For this review, take the finished solid that the model builds, in its own axes (mm). A direction names the side the tool comes from. Coordinates: 2 decimals unless noted, no trailing zeros. Order: outer loops, then holes, each group sorted by start corner. A loop starts at its lowest first (then second) coordinate and runs counter-clockwise, first axis right, second up.
from build123d import *

# Parameters (mm, degrees)
ESBO_O1_W                                           = 170
ESBO_O1_H                                           = 42
ESBO_O1_R                                           = 6
ESBO_O1_R_2                                         = 4
RESSALTO_EXTRUS_O1_DEPTH                            = 10
REBAIXO_PARA_PARAFUSO_COM_CABE_A_PANELA_D           = 3.4
REBAIXO_PARA_PARAFUSO_COM_CABE_A_PANELA_CBORE_D     = 7
REBAIXO_PARA_PARAFUSO_COM_CABE_A_PANELA_CBORE_DEPTH = 2.4
ESBO_O7_W                                           = 42.5
ESBO_O7_H                                           = 46.397828282
CORTE_EXTRUS_O2_DEPTH                               = 1.5
FILETE1_R                                           = 5


with BuildPart() as part:
    # Esboço1 → Ressalto-extrusão1 (new body)
    with BuildSketch(Plane(origin=(0, 0, 0), x_dir=(1, 0, 0), z_dir=(0, 1, 0))):
        Rectangle(ESBO_O1_W, ESBO_O1_H)
        with Locations(Location((-57.5, 0, 0), (0, 0, 270))):
            Circle(ESBO_O1_R, mode=Mode.SUBTRACT)
        with Locations(Location((57.5, 0, 0), (0, 0, 270))):
            Circle(ESBO_O1_R, mode=Mode.SUBTRACT)
        with Locations(Location((0, 0, 0), (0, 0, 270))):
            Circle(ESBO_O1_R_2, mode=Mode.SUBTRACT)
    extrude(amount=RESSALTO_EXTRUS_O1_DEPTH)

    # Esboço2 → Furo roscado de M51 (revolve, cut)
    with BuildSketch(Plane(origin=(85, 5, -1), x_dir=(0, 0, -1), z_dir=(0, 1, 0))):
        Polygon((0, 0), (0, 15.2618073), (2.1, 14), (2.1, 0), align=None)
    furo_roscado_de_m51 = revolve(axis=Axis((91.35, 5, -1), (-1, 0, 0)), mode=Mode.SUBTRACT)

    # Espelhar1: Furo roscado de M51 across plane
    add(furo_roscado_de_m51.mirror(Plane(origin=(0, 0, 0), x_dir=(0, 0, 1), z_dir=(1, 0, 0))), mode=Mode.SUBTRACT)

    # Rebaixo para parafuso com cabeça panela de M31 (through all)
    with Locations(Plane(origin=(0, 0, 0), x_dir=(-1, 0, 0), z_dir=(0, -1, 0))):
        with Locations((-15.5, 15.5), (15.5, 15.5), (-15.5, -15.5), (15.5, -15.5)):
            CounterBoreHole(REBAIXO_PARA_PARAFUSO_COM_CABE_A_PANELA_D / 2, REBAIXO_PARA_PARAFUSO_COM_CABE_A_PANELA_CBORE_D / 2, REBAIXO_PARA_PARAFUSO_COM_CABE_A_PANELA_CBORE_DEPTH)

    # Esboço7 → Corte-extrusão2 (cut)
    with BuildSketch(Plane(origin=(0, 10, 0), x_dir=(1, 0, 0), z_dir=(0, 1, 0))):
        with Locations((0, -0.001085859)):
            Rectangle(ESBO_O7_W, ESBO_O7_H)
    extrude(amount=-CORTE_EXTRUS_O2_DEPTH, mode=Mode.SUBTRACT)

    # Filete1
    filete1_edges = [part.edges().sort_by_distance(p)[0] for p in [
        (85, 5, 21),
        (-85, 5, 21),
        (-85, 5, -21),
        (85, 5, -21),
    ]]
    fillet(filete1_edges, radius=FILETE1_R)


solid = part.part
1. Clearance check with flat-ended pins moving along their axes: pin 1 Ø6.5 at (x, z) = (0, 0) entering from +Y; pin 2 Ø2.5 at (y, z) = (5, -1) entering from +X; pin 3 Ø4 at (x, z) = (-15.5, -15.5) entering from -Y; pin 4 Ø12.5 at (x, z) = (-1, 4.5) entering from +Y. State where each tip first meets the part, or that it passes through.
Answer below:
pin 1: passes through
pin 2: stops at x = 70.49
pin 3: stops at y = 2.4
pin 4: stops at y = 8.5
2. Machinability: for faces 1 (the face through (-84, 5, -19)), 2 (the face through (78.1, 7.05, -0.54)), 3 (the face through (12.16, 1.18, -16.55)), which of the approach directions +Z, -Z, +X, -X, +Y, -Y give a long, thin tool a straight path to every point of the face, cutting with its end or side? Answer none if there is none.
Answer below:
face 1: -Z, -X, +Y, -Y
face 2: +X
face 3: -Y
3. Take a section at C-C, the plane z = -10.5. Give the boundary of the cut face in (x, y).
Answer below:
outline: (-85, 0) - (85, 0) - (85, 10) - (21.25, 10) - (21.25, 8.5) - (-21.25, 8.5) - (-21.25, 10) - (-85, 10) - close
4. The part is to be moulded in two halves that separate along X. For faces 4 (the face through (-14.7, 5.5, -14)), 5 (the face through (-1, 5, -21)), 6 (the face through (-18.84, 1.18, -16.55)), 7 (the face through (-84, 5, 19)), say which applies: +X half, -X half, draft (parallel to the pull), parting line (faces both ways), or undercut.
Answer below:
face 4: undercut
face 5: draft
face 6: undercut
face 7: -X half
5. Take a section at B-B, the plane x = 57.5. Give the boundary of the cut face in (y, z).
Answer below:
outline: (0, -21) - (10, -21) - (10, -6) - (0, -6) - close; (0, 6) - (10, 6) - (10, 21) - (0, 21) - close
6. To check wall thickness, follow L1, parallel to X at y = 4.25, z = -15.5; L2, parallel to X at y = 1.6, z = -15.5; L3, parallel to Z at x = -15.5, y = 4.75. State the ranges of each line that lie inside material, in increasing order.
Answer below:
L1: x = -85 to -17.2, -13.8 to 13.8, 17.2 to 85
L2: x = -85 to -19, -12 to 12, 19 to 85
L3: z = -21 to -17.2, -13.8 to 13.8, 17.2 to 21
7. Take a section at A-A, the plane x = -15.5. Give the boundary of the cut face in (y, z).
Answer below:
outline: (0, -21) - (8.5, -21) - (8.5, -17.2) - (2.4, -17.2) - (2.4, -19) - (0, -19) - close; (0, -12) - (2.4, -12) - (2.4, -13.8) - (8.5, -13.8) - (8.5, 13.8) - (2.4, 13.8) - (2.4, 12) - (0, 12) - close; (0, 19) - (2.4, 19) - (2.4, 17.2) - (8.5, 17.2) - (8.5, 21) - (0, 21) - close
